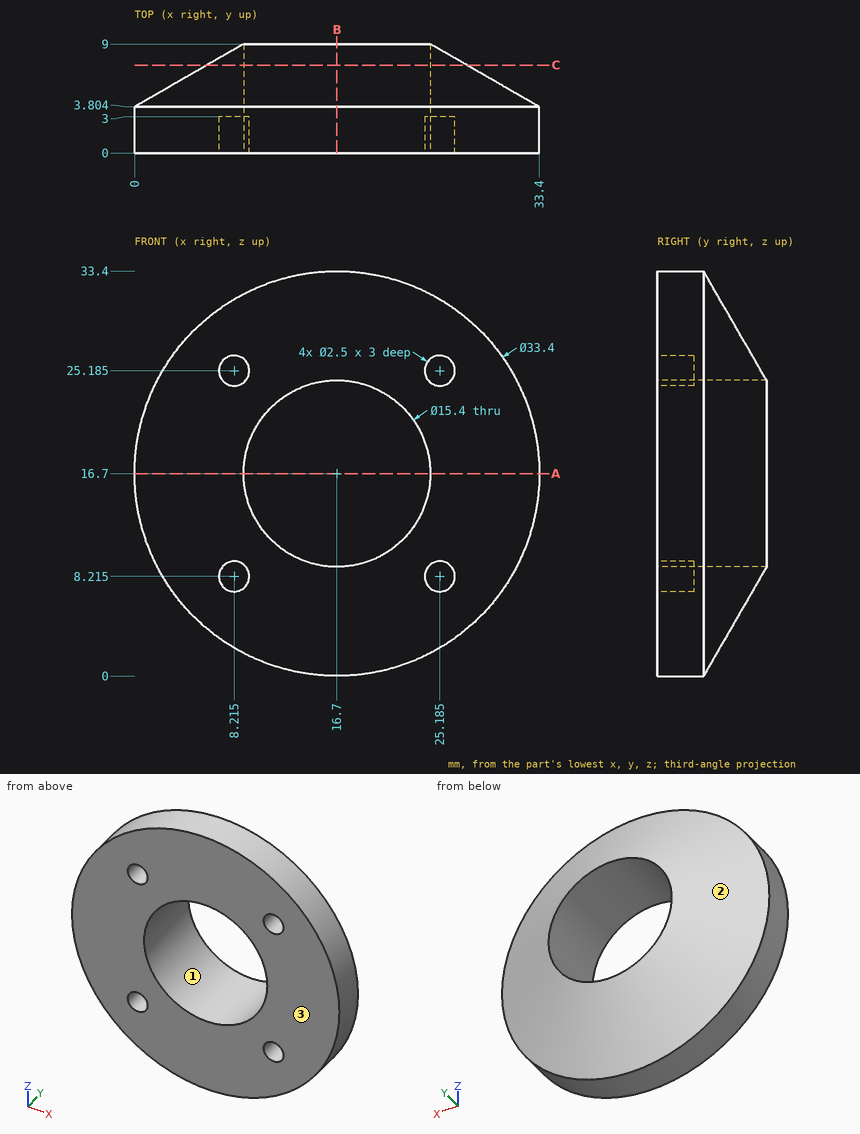
Source: three-view drawing plus pictorial views. Frame: mm from the lowest corner of the part. Coordinates: 2 decimals unless noted, no trailing zeros. Loops run counter-clockwise (first coordinate to the right, second up) from the corner with the lowest first, then second, coordinate; pieces in that order, holes last. Notation, with made-up numbers: (-32.75, -36) -> (26.25, -36) arc R14 cw to (26.25, -24) -> close; hole circle Ø8 at (58.25, 27). An arc over 180 degrees is marked (long way). One line per item, written item: value.
(1) Cut plane C-C (y = 7.25). Output: boundary loops of the cut face in (x, z).
Answer below:
outline: circle Ø21.46 at (16.7, 16.7); hole circle Ø15.4 at (16.7, 16.7)
(2) Draft query along Z for the marked faces 1, 2 and 3. Return one class per face: pulls with the +Z half, pulls with the -Z half, needs draft (parallel to the pull), parting line crosses it, or undercut.
Answer below:
face 1: undercut
face 2: parting line crosses it
face 3: needs draft
(3) Pin query (flat end, axial travel): pin 1 Ø1.2 at (x, z) = (8.5, 25) entering from -Y; pin 2 Ø1.2 at (x, z) = (25.5, 7.5) entering from -Y; pin 3 Ø5 at (x, y) = (6.5, 4) entering from +Z (1 decimal); pin 4 Ø2 at (x, y) = (21, 6.5) entering from +Z. Return the tip coordinate at first contact, or that it passes through.
Answer below:
pin 1: stops at y = 3
pin 2: stops at y = 0
pin 3: stops at z = 31.5
pin 4: stops at z = 29.8
(4) Cut plane A-A (z = 16.7). Output: boundary loops of the cut face in (x, y), then the cut area to 3 significant figures.
Answer below:
outline: (0, 0) -> (9, 0) -> (9, 9) -> (0, 3.8) -> close; (24.4, 0) -> (33.4, 0) -> (33.4, 3.8) -> (24.4, 9) -> close
area: 115 mm2
(5) Cut plane B-B (x = 16.7). Output: boundary loops of the cut face in (y, z), then the cut area to 3 significant figures.
Answer below:
outline: (0, 0) -> (3.8, 0) -> (9, 9) -> (0, 9) -> close; (0, 24.4) -> (9, 24.4) -> (3.8, 33.4) -> (0, 33.4) -> close
area: 115 mm2
(6) Ray query, line 1 along Z through (x, y) = (16.5, 2); line 2 along X through (y, z) = (7, 13) (1 decimal); line 3 along X through (y, z) = (7, 16.7) (1 decimal). Return the intervals inside material, ascending.
Answer below:
line 1: z = 0 to 9, 24.4 to 33.4
line 2: x = 6.2 to 9.9, 23.5 to 27.2
line 3: x = 5.5 to 9, 24.4 to 27.9
